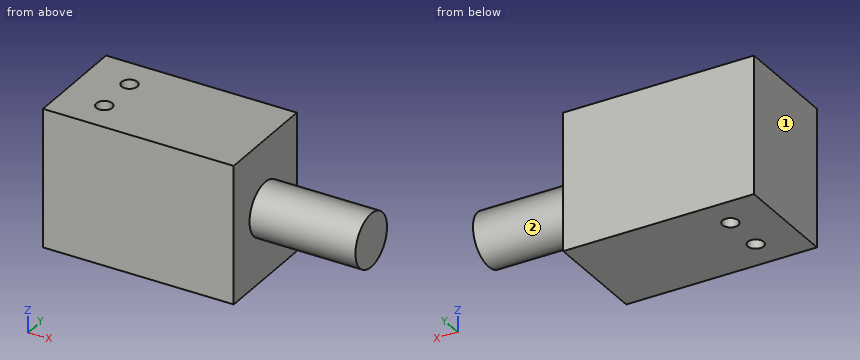
from build123d import *

# Parameters (mm, degrees)
SKETCH119_W     = 36
SKETCH119_H     = 20
PAD083_DEPTH    = 26
SKETCH120_R     = 5
PAD084_DEPTH    = 20
SKETCH137_R     = 1.5
POCKET108_DEPTH = 26.001


with BuildPart() as part:
    # Sketch119 → Pad083 (new body)
    with BuildSketch(Plane.XY):
        with Locations((-46, 0)):
            Rectangle(SKETCH119_W, SKETCH119_H)
    extrude(amount=PAD083_DEPTH)

    # Sketch120 (on Face2 of Pad083) → Pad084 (join)
    with BuildSketch(Plane.YZ.offset(-28)):
        with Locations((0, 13)):
            Circle(SKETCH120_R)
    extrude(amount=PAD084_DEPTH)

    # Sketch137 (on Face5 of Pad084) → Pocket108 (cut, through all)
    with BuildSketch(Plane.XY.offset(26)):
        with Locations((-56, 4)):
            Circle(SKETCH137_R)
        with Locations((-56, -4)):
            Circle(SKETCH137_R)
    extrude(amount=-POCKET108_DEPTH, mode=Mode.SUBTRACT)


with BuildPart() as part_1:
    # Body049 placement: moved
    add(part.part.moved(Location((-1, 0, -15))))


solid = part_1.part
Geometry check sheet. Reference: the model listing, model coordinates, mm. Face numbers are marked on the shaded views. A direction names the side the tool comes from. Coordinates: 2 decimals unless noted, no trailing zeros. Write each loop counter-clockwise with the first axis right and the second up, starting at its lowest first coordinate (ties: lowest second). Pieces come first, ordered by that corner, then holes. Notation, with made-up numbers: (27, -7.75) -> (66, -7.75) arc R13 cw to (66, 4.25) -> close; hole circle Ø1 at (-12.5, 20.5). An arc over 180 degrees is marked (long way). One line per question, with ' | ' between items.
1. Depth check by flat-ended pin: pin 1 Ø3 at (x, y) = (-19, -4) entering from -Z. Enter the tip coordinate at first touch or a pass-through.
Answers:
pin 1: stops at z = -6.33
2. Set-up check for the marked faces 1 and 2: record each of +Z, -Z, +X, -X, +Y, -Y from which the full face is reachable in a straight line by a thin tool's end or side.
Answers:
face 1: +Z, -Z, -X, +Y, -Y | face 2: +X
3. Cross-section at B-B on z = -2. Record the cut outline in (x, y), and give its area (3 significant figures).
Answers:
outline: (-65, -10) -> (-29, -10) -> (-29, -5) -> (-9, -5) -> (-9, 5) -> (-29, 5) -> (-29, 10) -> (-65, 10) -> close; hole circle Ø3 at (-57, -4); hole circle Ø3 at (-57, 4) | area: 906 mm²
4. Cross-section at D-D on z = 5.25. Record the cut outline in (x, y).
Answers:
outline: (-65, -10) -> (-29, -10) -> (-29, 10) -> (-65, 10) -> close; hole circle Ø3 at (-57, -4); hole circle Ø3 at (-57, 4)
5. Cross-section at A-A on y = 4. Record the cut outline in (x, z), and give its area (3 significant figures).
Answers:
outline: (-65, -15) -> (-58.5, -15) -> (-58.5, 11) -> (-65, 11) -> close; (-55.5, -15) -> (-29, -15) -> (-29, -5) -> (-9, -5) -> (-9, 1) -> (-29, 1) -> (-29, 11) -> (-55.5, 11) -> close | area: 978 mm²
6. Cross-section at C-C on y = 0. Record the cut outline in (x, z), and give its area (3 significant figures).
Answers:
outline: (-65, -15) -> (-29, -15) -> (-29, -7) -> (-9, -7) -> (-9, 3) -> (-29, 3) -> (-29, 11) -> (-65, 11) -> close | area: 1,140 mm²
7. Thickness scan on probe 1 along Y at (x, z) = (-57, -4.25); probe 2 along Y at (x, z) = (-12, -1.75); probe 3 along X at (y, z) = (-6.75, 3.25). Record the ranges inside material, lowest first. Write a range as from..to.
Answers:
probe 1: y = -10..-5.5, -2.5..2.5, 5.5..10 | probe 2: y = -4.99..4.99 | probe 3: x = -65..-29
